```python
from build123d import *

# Parameters (mm, degrees)
SKETCH1_W           = 100
SKETCH1_H           = 80
BOSS_EXTRUDE1_DEPTH = 40
CUT_EXTRUDE1_REACH  = 77.498
SKETCH2_R           = 7.5
SKETCH2_R_2         = 10.5
CUT_EXTRUDE2_REACH  = 77.498
SKETCH3_W           = 100
SKETCH3_H           = 20
CUT_EXTRUDE4_REACH  = 77.498
SKETCH5_W           = 50
SKETCH5_H           = 25
FILLET1_R           = 10
FILLET2_R           = 10
FILLET3_R           = 10
FILLET4_R           = 10
SKETCH6_W           = 50
SKETCH6_H           = 40
BOSS_EXTRUDE2_DEPTH = 20
SKETCH4_R           = 3
CUT_EXTRUDE5_DEPTH  = 20


with BuildPart() as part:
    # Sketch1 → Boss-Extrude1 (new body)
    with BuildSketch(Plane.XY):
        Rectangle(SKETCH1_W, SKETCH1_H)
    extrude(amount=BOSS_EXTRUDE1_DEPTH)

    # Sketch2 → Cut-Extrude1 (cut, up to next)
    with BuildSketch(Plane.XY.offset(40), mode=Mode.PRIVATE) as cut_extrude1_sk1:
        Circle(SKETCH2_R)
    cut_extrude1_tool1 = extrude(cut_extrude1_sk1.sketch, amount=-CUT_EXTRUDE1_REACH, mode=Mode.PRIVATE) & part.part
    # Sketch2 → Cut-Extrude1 (cut, up to next)
    with BuildSketch(Plane.XY.offset(40), mode=Mode.PRIVATE) as cut_extrude1_sk2:
        with Locations((-35, 0)):
            Circle(SKETCH2_R_2)
    cut_extrude1_tool2 = extrude(cut_extrude1_sk2.sketch, amount=-CUT_EXTRUDE1_REACH, mode=Mode.PRIVATE) & part.part
    # Sketch2 → Cut-Extrude1 (cut, up to next)
    with BuildSketch(Plane.XY.offset(40), mode=Mode.PRIVATE) as cut_extrude1_sk3:
        with Locations((35, 0)):
            Circle(SKETCH2_R_2)
    cut_extrude1_tool3 = extrude(cut_extrude1_sk3.sketch, amount=-CUT_EXTRUDE1_REACH, mode=Mode.PRIVATE) & part.part
    add(cut_extrude1_tool1.solids().sort_by_distance((0, 0, 40))[0], mode=Mode.SUBTRACT)
    add(cut_extrude1_tool2.solids().sort_by_distance((-35, 0, 40))[0], mode=Mode.SUBTRACT)
    add(cut_extrude1_tool3.solids().sort_by_distance((35, 0, 40))[0], mode=Mode.SUBTRACT)

    # Sketch3 → Cut-Extrude2 (cut, up to next)
    with BuildSketch(Plane.XY.offset(40), mode=Mode.PRIVATE) as cut_extrude2_sk1:
        with Locations((0, 30)):
            Rectangle(SKETCH3_W, SKETCH3_H)
    cut_extrude2_tool1 = extrude(cut_extrude2_sk1.sketch, amount=-CUT_EXTRUDE2_REACH, mode=Mode.PRIVATE) & part.part
    add(cut_extrude2_tool1.solids().sort_by_distance((0, 30, 40))[0], mode=Mode.SUBTRACT)

    # Sketch5 → Cut-Extrude4 (cut, up to next)
    with BuildSketch(Plane(origin=(0, 0, 0), x_dir=(-1, 0, 0), z_dir=(0, 0, -1)), mode=Mode.PRIVATE) as cut_extrude4_sk1:
        with Locations((25, -27.5)):
            Rectangle(SKETCH5_W, SKETCH5_H)
    cut_extrude4_tool1 = extrude(cut_extrude4_sk1.sketch, amount=-CUT_EXTRUDE4_REACH, mode=Mode.PRIVATE) & part.part
    add(cut_extrude4_tool1.solids().sort_by_distance((-25, -27.5, 0))[0], mode=Mode.SUBTRACT)

    # Fillet1
    fillet1_edges = [part.edges().sort_by_distance(p)[0] for p in [
        (0, -15, 20),
    ]]
    fillet(fillet1_edges, radius=FILLET1_R)

    # Fillet2
    fillet2_edges = [part.edges().sort_by_distance(p)[0] for p in [
        (-50, -15, 20),
    ]]
    fillet(fillet2_edges, radius=FILLET2_R)

    # Fillet3
    fillet3_edges = [part.edges().sort_by_distance(p)[0] for p in [
        (-50, 20, 20),
    ]]
    fillet(fillet3_edges, radius=FILLET3_R)

    # Fillet4
    fillet4_edges = [part.edges().sort_by_distance(p)[0] for p in [
        (50, 20, 20),
    ]]
    fillet(fillet4_edges, radius=FILLET4_R)

    # Sketch6 → Boss-Extrude2 (add)
    with BuildSketch(Plane.XZ.offset(40)):
        with Locations((25, 20)):
            Rectangle(SKETCH6_W, SKETCH6_H)
    extrude(amount=BOSS_EXTRUDE2_DEPTH)

    # Sketch4 → Cut-Extrude5 (cut, symmetric)
    with BuildSketch(Plane.XZ.offset(40)):
        with Locations(Location((16, 20, 0), (0, 0, 180))):
            Circle(SKETCH4_R)
        with Locations(Location((36, 20, 0), (0, 0, 180))):
            Circle(SKETCH4_R)
    extrude(amount=CUT_EXTRUDE5_DEPTH, both=True, mode=Mode.SUBTRACT)


solid = part.part
```
Geometry check sheet. Reference: the model listing, model coordinates, mm. A direction names the side the tool comes from. Give positions to 0.01 mm unless a question says otherwise; leave off trailing zeros. Write each loop counter-clockwise with the first axis right and the second up, starting at its lowest first coordinate (ties: lowest second). Pieces come first, ordered by that corner, then holes. Notation, with made-up numbers: (-18.5, 83) - (39.5, 83) arc R22 cw to (39.5, 91) - close; hole circle Ø4 at (-36, 64.5). An arc over 180 degrees is marked (long way). Use a Markdown table: item, result.
Q1. Draft check along Y on faces 1 (the face through (-46.99, -12.15, 20.28)), 2 (the face through (-7.493, 0.33, 20.28)), 3 (the face through (-45.49, 0.46, 20.28)), 4 (the face through (10, -11, 40)). Enter one of: pulls with the +Y half, pulls with the -Y half, needs draft (parallel to the pull), parting line crosses it, or undercut.
Computed:
| item | result |
|---|---|
| face 1 | pulls with the -Y half |
| face 2 | undercut |
| face 3 | undercut |
| face 4 | needs draft |
Q2. Section check C-C, the plane x = -35. Enter the section's corners in (y, z), then the cut area to 3 significant figures.
Computed:
| item | result |
|---|---|
| outline | (-15, 0) - (-10.5, 0) - (-10.5, 40) - (-15, 40) - close; (10.5, 0) - (20, 0) - (20, 40) - (10.5, 40) - close |
| area | 560 mm² |
Q3. Section check A-A, the plane z = 20. Enter the section's corners in (x, y), then the cut area to 3 significant figures.
Computed:
| item | result |
|---|---|
| outline | (-50, -5) arc R10 ccw to (-40, -15) - (-10, -15) arc R10 cw to (0, -25) - (0, -60) - (13, -60) - (13, -20) - (19, -20) - (19, -60) - (33, -60) - (33, -20) - (39, -20) - (39, -60) - (50, -60) - (50, 10) arc R10 ccw to (40, 20) - (-40, 20) arc R10 ccw to (-50, 10) - close; hole circle Ø21 at (-35, 0); hole circle Ø15 at (0, 0); hole circle Ø21 at (35, 0) |
| area | 4,360 mm² |
Q4. Set-up check for faces 5 (the face through (39, -40, 20)), 6 (the face through (-1, 20, 20)), 7 (the face through (0, -42, 20)): record each of +Z, -Z, +X, -X, +Y, -Y from which the full face is reachable in a straight line by a thin tool's end or side.
Computed:
| item | result |
|---|---|
| face 5 | -Y |
| face 6 | +Z, -Z, +X, -X, +Y |
| face 7 | +Z, -Z, -X, -Y |
Q5. Go/stop test with flat-tipped pins: P1, Ø10, axis at x = -8, y = -50.5, coming from the +Z side; P2, Ø6.5, axis at x = 34.5, z = 19, coming from the -Y side; P3, Ø8, axis at y = -32, z = 5.5, coming from the -X side; P4, Ø9, axis at x = -23, z = 16, coming from the -Y side. Record where each tip stops, or that it passes through.
Computed:
| item | result |
|---|---|
| P1 | passes through |
| P2 | stops at y = -60 |
| P3 | stops at x = 0 |
| P4 | stops at y = -15 |
Q6. Thickness scan on L1, parallel to X at y = -29, z = 20; L2, parallel to Y at x = -35, z = 16.5; L3, parallel to Y at x = 35.5, z = 14.5. Record the ranges inside material, lowest first. Write a range as [from, to].
Computed:
| item | result |
|---|---|
| L1 | x = [0, 13], [19, 33], [39, 50] |
| L2 | y = [-15, -10.5], [10.5, 20] |
| L3 | y = [-60, -10.49], [10.49, 20] |
Q7. Section check B-B, the plane y = 0. Enter the section's corners in (x, z), then the cut area to 3 significant figures.
Computed:
| item | result |
|---|---|
| outline | (-50, 0) - (-45.5, 0) - (-45.5, 40) - (-50, 40) - close; (-24.5, 0) - (-7.5, 0) - (-7.5, 40) - (-24.5, 40) - close; (7.5, 0) - (24.5, 0) - (24.5, 40) - (7.5, 40) - close; (45.5, 0) - (50, 0) - (50, 40) - (45.5, 40) - close |
| area | 1,720 mm² |
Q8. Section check D-D, the plane x = 16. Enter the section's corners in (y, z), then the cut area to 3 significant figures.
Computed:
| item | result |
|---|---|
| outline | (-60, 0) - (20, 0) - (20, 40) - (-60, 40) - (-60, 23) - (-20, 23) - (-20, 17) - (-60, 17) - close |
| area | 2,960 mm² |
